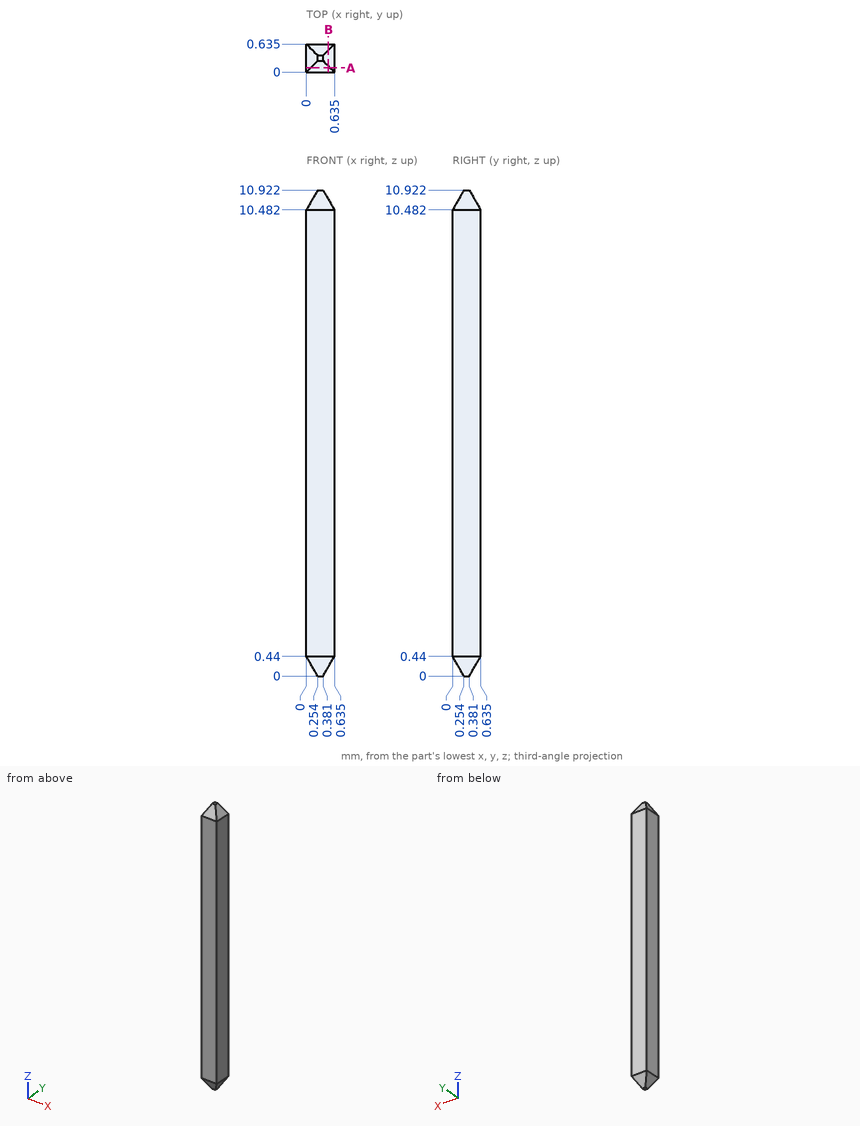
Source: three-view drawing plus pictorial views. Frame: mm from the lowest corner of the part. Round coordinates to 2 decimals unless told otherwise and drop trailing zeros. Loops run counter-clockwise (first coordinate to the right, second up) from the corner with the lowest first, then second, coordinate; pieces in that order, holes last. Notation, with made-up numbers: M 60.25,-12 L 86.25,-12 A4 ccw 86.25,-7 Z; hole C 9.5,74 d4. An arc over 180 degrees is marked long. Put each result on its own line as item: value.
(1) Ray query, line 1 (Z direction, x = 0.2, y = 0.25); line 2 (Z direction, x = 0.2, y = 0.55). Return the intervals inside material, ascending. Write a range as [from, to].
Solutions:
line 1: [0.09, 10.83]
line 2: [0.29, 10.63]
(2) Section B-B, the plane x = 0.5. Return loops of the section in (y, z) (3 decimals), and give its area (3 significant figures).
Solutions:
outline: M 0,0.44 L 0.135,0.206 L 0.5,0.206 L 0.635,0.44 L 0.635,10.482 L 0.5,10.716 L 0.135,10.716 L 0,10.482 Z
area: 6.61 mm²
(3) Section A-A, the plane y = 0.1. Return loops of the section in (x, z) (3 decimals), and give its area (3 significant figures).
Solutions:
outline: M 0,0.44 L 0.1,0.267 L 0.535,0.267 L 0.635,0.44 L 0.635,10.482 L 0.535,10.655 L 0.1,10.655 L 0,10.482 Z
area: 6.56 mm²
